```python
from build123d import *

# Parameters (mm, degrees)
RESSALTO_EXTRUS_O1_DEPTH = 6
ESBO_O7_W                = 6
ESBO_O7_H                = 39
CORTE_EXTRUS_O5_DEPTH    = 441.818556778
ESBO_O2_W                = 98
ESBO_O2_H                = 88
CORTE_EXTRUS_O1_DEPTH    = 10
FILETE2_R                = 12
CORTE_EXTRUS_O3_DEPTH    = 441.818556778
ESBO_O6_W                = 30
ESBO_O6_H                = 20
CORTE_EXTRUS_O4_DEPTH    = 441.818556778
FILETE3_START            = -1
FILETE3_DEPTH            = 8
FILETE3_2_DEPTH          = 6
ESBO_O8_W                = 6
ESBO_O8_H                = 34
RESSALTO_EXTRUS_O2_DEPTH = 31.4
ESBO_O9_W                = 25.4
ESBO_O9_H                = 55
RESSALTO_EXTRUS_O3_DEPTH = 6
CHANFRO1_SIZE            = 3
ESBO_O10_R               = 3.257801974
ESBO_O10_R_2             = 3
ESBO_O10_R_3             = 3.08509383
CORTE_EXTRUS_O6_DEPTH    = 463.399134947
FILETE4_R                = 5
ESBO_O11_W               = 402.172610053
ESBO_O11_H               = 13.658923547
CORTE_EXTRUS_O7_DEPTH    = 463.399134947
FILETE5_R                = 5


with BuildPart() as part:
    # Esboço1 → Ressalto-extrusão1 (new body)
    with BuildSketch(Plane.XY):
        Polygon((0, 94), (0, 238), (365, 238), (365, 94), (371, 94), (371, 0), (365, 0), (0, 0), (-6, 0), (-6, 94), align=None)
    extrude(amount=RESSALTO_EXTRUS_O1_DEPTH)

    # Esboço7 → Corte-extrusão5 (cut, through all)
    with BuildSketch(Plane.XY.offset(6)):
        with Locations((368, 19.5)):
            Rectangle(ESBO_O7_W, ESBO_O7_H)
        with Locations((-3, 19.5)):
            Rectangle(ESBO_O7_W, ESBO_O7_H)
    extrude(amount=-CORTE_EXTRUS_O5_DEPTH, mode=Mode.SUBTRACT)

    # Esboço2 → Corte-extrusão1 (cut)
    with BuildSketch(Plane.XY.offset(6)):
        with Locations((64, 144)):
            Rectangle(ESBO_O2_W, ESBO_O2_H)
        with Locations((301, 144)):
            Rectangle(ESBO_O2_W, ESBO_O2_H)
    extrude(amount=-CORTE_EXTRUS_O1_DEPTH, mode=Mode.SUBTRACT)

    # Filete2
    filete2_edges = [part.edges().sort_by_distance(p)[0] for p in [
        (15, 100, 3),
        (15, 188, 3),
        (113, 188, 3),
        (113, 100, 3),
        (350, 188, 3),
        (350, 100, 3),
        (252, 100, 3),
        (252, 188, 3),
    ]]
    fillet(filete2_edges, radius=FILETE2_R)

    # Esboço5 → Corte-extrusão3 (cut, through all)
    with BuildSketch(Plane.XY.offset(6)):
        with BuildLine():
            Line((183.428625358, 61.017420231), (160.787066224, 38.375861098))
            ThreePointArc((160.787066224, 38.375861098), (157.965710167, 37.207217155), (155.14435411, 38.375861098))
            Line((155.14435411, 38.375861098), (155.130211974, 38.390003233))
            ThreePointArc((155.130211974, 38.390003233), (153.961568031, 41.21135929), (155.130211974, 44.032715347))
            Line((155.130211974, 44.032715347), (177.771771108, 66.674274481))
            ThreePointArc((177.771771108, 66.674274481), (180.593127165, 67.842918424), (183.414483222, 66.674274481))
            Line((183.414483222, 66.674274481), (183.428625358, 66.660132345))
            ThreePointArc((183.428625358, 66.660132345), (184.597269301, 63.838776288), (183.428625358, 61.017420231))
        make_face()
        with BuildLine():
            Line((177.771771108, 82.046857483), (177.757628972, 82.032715347))
            ThreePointArc((177.757628972, 82.032715347), (176.588985029, 79.21135929), (177.757628972, 76.390003233))
            Line((177.757628972, 76.390003233), (200.399188106, 53.7484441))
            ThreePointArc((200.399188106, 53.7484441), (203.220544163, 52.579800157), (206.04190022, 53.7484441))
            Line((206.04190022, 53.7484441), (206.056042356, 53.762586235))
            ThreePointArc((206.056042356, 53.762586235), (207.224686299, 56.583942292), (206.056042356, 59.405298349))
            Line((206.056042356, 59.405298349), (183.414483222, 82.046857483))
            ThreePointArc((183.414483222, 82.046857483), (180.593127165, 83.215501426), (177.771771108, 82.046857483))
        make_face()
        with BuildLine():
            Line((183.428625358, 99.017420231), (160.787066224, 76.375861098))
            ThreePointArc((160.787066224, 76.375861098), (157.965710167, 75.207217155), (155.14435411, 76.375861098))
            Line((155.14435411, 76.375861098), (155.130211974, 76.390003233))
            ThreePointArc((155.130211974, 76.390003233), (153.961568031, 79.21135929), (155.130211974, 82.032715347))
            Line((155.130211974, 82.032715347), (177.771771108, 104.674274481))
            ThreePointArc((177.771771108, 104.674274481), (180.593127165, 105.842918424), (183.414483222, 104.674274481))
            Line((183.414483222, 104.674274481), (183.428625358, 104.660132345))
            ThreePointArc((183.428625358, 104.660132345), (184.597269301, 101.838776288), (183.428625358, 99.017420231))
        make_face()
        with BuildLine():
            Line((177.771771108, 120.046857483), (177.757628972, 120.032715347))
            ThreePointArc((177.757628972, 120.032715347), (176.588985029, 117.21135929), (177.757628972, 114.390003233))
            Line((177.757628972, 114.390003233), (200.399188106, 91.7484441))
            ThreePointArc((200.399188106, 91.7484441), (203.220544163, 90.579800157), (206.04190022, 91.7484441))
            Line((206.04190022, 91.7484441), (206.056042356, 91.762586235))
            ThreePointArc((206.056042356, 91.762586235), (207.224686299, 94.583942292), (206.056042356, 97.405298349))
            Line((206.056042356, 97.405298349), (183.414483222, 120.046857483))
            ThreePointArc((183.414483222, 120.046857483), (180.593127165, 121.215501426), (177.771771108, 120.046857483))
        make_face()
        with BuildLine():
            Line((183.428625358, 137.017420231), (160.787066224, 114.375861098))
            ThreePointArc((160.787066224, 114.375861098), (157.965710167, 113.207217155), (155.14435411, 114.375861098))
            Line((155.14435411, 114.375861098), (155.130211974, 114.390003233))
            ThreePointArc((155.130211974, 114.390003233), (153.961568031, 117.21135929), (155.130211974, 120.032715347))
            Line((155.130211974, 120.032715347), (177.771771108, 142.674274481))
            ThreePointArc((177.771771108, 142.674274481), (180.593127165, 143.842918424), (183.414483222, 142.674274481))
            Line((183.414483222, 142.674274481), (183.428625358, 142.660132345))
            ThreePointArc((183.428625358, 142.660132345), (184.597269301, 139.838776288), (183.428625358, 137.017420231))
        make_face()
        with BuildLine():
            Line((177.771771108, 158.046857483), (177.757628972, 158.032715347))
            ThreePointArc((177.757628972, 158.032715347), (176.588985029, 155.21135929), (177.757628972, 152.390003233))
            Line((177.757628972, 152.390003233), (200.399188106, 129.7484441))
            ThreePointArc((200.399188106, 129.7484441), (203.220544163, 128.579800157), (206.04190022, 129.7484441))
            Line((206.04190022, 129.7484441), (206.056042356, 129.762586235))
            ThreePointArc((206.056042356, 129.762586235), (207.224686299, 132.583942292), (206.056042356, 135.405298349))
            Line((206.056042356, 135.405298349), (183.414483222, 158.046857483))
            ThreePointArc((183.414483222, 158.046857483), (180.593127165, 159.215501426), (177.771771108, 158.046857483))
        make_face()
        with BuildLine():
            Line((183.428625358, 175.017420231), (160.787066224, 152.375861098))
            ThreePointArc((160.787066224, 152.375861098), (157.965710167, 151.207217155), (155.14435411, 152.375861098))
            Line((155.14435411, 152.375861098), (155.130211974, 152.390003233))
            ThreePointArc((155.130211974, 152.390003233), (153.961568031, 155.21135929), (155.130211974, 158.032715347))
            Line((155.130211974, 158.032715347), (177.771771108, 180.674274481))
            ThreePointArc((177.771771108, 180.674274481), (180.593127165, 181.842918424), (183.414483222, 180.674274481))
            Line((183.414483222, 180.674274481), (183.428625358, 180.660132345))
            ThreePointArc((183.428625358, 180.660132345), (184.597269301, 177.838776288), (183.428625358, 175.017420231))
        make_face()
    extrude(amount=-CORTE_EXTRUS_O3_DEPTH, mode=Mode.SUBTRACT)

    # Esboço6 → Corte-extrusão4 (cut, through all)
    with BuildSketch(Plane.XY.offset(6)):
        with Locations((107.5, 10)):
            Rectangle(ESBO_O6_W, ESBO_O6_H)
        with Locations((257.5, 10)):
            Rectangle(ESBO_O6_W, ESBO_O6_H)
    extrude(amount=-CORTE_EXTRUS_O4_DEPTH, mode=Mode.SUBTRACT)

    # Filete3: read off the stored shape, not the designer's step
    # Filete3 outline → Filete3 (cut)
    with BuildSketch(Plane.XY.offset(FILETE3_START)):
        with BuildLine():
            ThreePointArc((282.5, 0), (275.428932188, 2.928932188), (272.5, 10))
            Line((272.5, 10), (272.5, 0))
            Line((272.5, 0), (282.5, 0))
        make_face()
        with BuildLine():
            Line((92.5, 0), (92.5, 10))
            ThreePointArc((92.5, 10), (89.571067812, 2.928932188), (82.5, 0))
            Line((82.5, 0), (92.5, 0))
        make_face()
        with BuildLine():
            Line((122.5, 0), (132.5, 0))
            ThreePointArc((132.5, 0), (125.428932188, 2.928932188), (122.5, 10))
            Line((122.5, 10), (122.5, 0))
        make_face()
        with BuildLine():
            Line((242.5, 0), (242.5, 10))
            ThreePointArc((242.5, 10), (239.571067812, 2.928932188), (232.5, 0))
            Line((232.5, 0), (242.5, 0))
        make_face()
    extrude(amount=FILETE3_DEPTH, mode=Mode.SUBTRACT)

    # Filete3 2 outline → Filete3 2 (add)
    with BuildSketch(Plane.XY):
        with BuildLine():
            Line((272.5, 20), (262.5, 20))
            ThreePointArc((262.5, 20), (269.571067812, 17.071067812), (272.5, 10))
            Line((272.5, 10), (272.5, 20))
        make_face()
        with BuildLine():
            ThreePointArc((92.5, 10), (95.428932188, 17.071067812), (102.5, 20))
            Line((102.5, 20), (92.5, 20))
            Line((92.5, 20), (92.5, 10))
        make_face()
        with BuildLine():
            ThreePointArc((112.5, 20), (119.571067812, 17.071067812), (122.5, 10))
            Line((122.5, 10), (122.5, 20))
            Line((122.5, 20), (112.5, 20))
        make_face()
        with BuildLine():
            ThreePointArc((242.5, 10), (245.428932188, 17.071067812), (252.5, 20))
            Line((252.5, 20), (242.5, 20))
            Line((242.5, 20), (242.5, 10))
        make_face()
    extrude(amount=FILETE3_2_DEPTH)

    # Esboço8 → Ressalto-extrusão2 (add)
    with BuildSketch(Plane(origin=(365, 0, 0), x_dir=(0, 0, -1), z_dir=(1, 0, 0))):
        with Locations((-3, 207.827931833)):
            Rectangle(ESBO_O8_W, ESBO_O8_H)
    ressalto_extrus_o2 = extrude(amount=RESSALTO_EXTRUS_O2_DEPTH)

    # Espelhar1: Ressalto-extrusão2 across plane
    add(ressalto_extrus_o2.mirror(Plane.ZY.offset(-182.5)))

    # Esboço9 → Ressalto-extrusão3 (add, through all)
    with BuildSketch(Plane.XY.offset(6)):
        with Locations((383.7, 66.5)):
            Rectangle(ESBO_O9_W, ESBO_O9_H)
        with Locations((-18.7, 66.5)):
            Rectangle(ESBO_O9_W, ESBO_O9_H)
    extrude(amount=-RESSALTO_EXTRUS_O3_DEPTH)

    # Chanfro1
    chanfro1_edges = [part.edges().sort_by_distance(p)[0] for p in [
        (396.4, 224.827931833, 3),
        (396.4, 190.827931833, 3),
        (-31.4, 224.827931833, 3),
        (-31.4, 190.827931833, 3),
        (396.4, 94, 3),
        (396.4, 39, 3),
        (-31.4, 39, 3),
        (-31.4, 94, 3),
    ]]
    chamfer(chanfro1_edges, length=CHANFRO1_SIZE)

    # Esboço10 → Corte-extrusão6 (cut, through all)
    with BuildSketch(Plane.XY.offset(6)):
        with Locations((385.342976088, 207.820691694)):
            Circle(ESBO_O10_R)
        with Locations((385.3, 83.913025663)):
            Circle(ESBO_O10_R_2)
        with Locations((385.3, 49.913025663)):
            Circle(ESBO_O10_R_3)
        with Locations(Location((-20.3, 49.913025663, 0), (0, 0, 180))):
            Circle(ESBO_O10_R_3)
        with Locations(Location((-20.3, 83.913025663, 0), (0, 0, 180))):
            Circle(ESBO_O10_R_2)
        with Locations(Location((-20.342976088, 207.820691694, 0), (0, 0, 180))):
            Circle(ESBO_O10_R)
    extrude(amount=-CORTE_EXTRUS_O6_DEPTH, mode=Mode.SUBTRACT)

    # Filete4
    filete4_edges = [part.edges().sort_by_distance(p)[0] for p in [
        (365, 0, 3),
        (0, 0, 3),
    ]]
    fillet(filete4_edges, radius=FILETE4_R)

    # Esboço11 → Corte-extrusão7 (cut, through all)
    with BuildSketch(Plane.XY.offset(6)):
        with Locations((201.086305027, 2.170538226)):
            Rectangle(ESBO_O11_W, ESBO_O11_H)
    extrude(amount=-CORTE_EXTRUS_O7_DEPTH, mode=Mode.SUBTRACT)

    # Filete5
    filete5_edges = [part.edges().sort_by_distance(p)[0] for p in [
        (0, 9, 3),
        (122.550125629, 9, 3),
        (92.449874371, 9, 3),
        (242.449874371, 9, 3),
        (272.550125629, 9, 3),
        (365, 9, 3),
    ]]
    fillet(filete5_edges, radius=FILETE5_R)


solid = part.part
```
CAD build for the part. Positions are in the model's coordinates, mm. A direction names the side the tool comes from. Coordinates: 2 decimals unless noted, no trailing zeros. Order: outer loops, then holes, each group sorted by start corner. A loop starts at its lowest first (then second) coordinate and runs counter-clockwise, first axis right, second up. Notation, with made-up numbers: M 18.25,-29.5 L 64.25,-29.5 A17 ccw 64.25,-18.5 Z; hole C 50,62 d1. An arc over 180 degrees is marked long. Write each question's results on one line, items separated by ' | '. Start each with the question number.
Q1. Drill centre lines: probe 1 along Y at (x, z) = (277, 5.25); probe 2 along X at (y, z) = (102.5, 1.5); probe 3 along Y at (x, z) = (385.3, 1.55). Where is each one in solid material? Low to high. Write a range as from..to.
Q2. Cut at B-B (z = 3.75). Count the separate pieces of the cut face and the enclosed holes in it, then the cut area to 3 significant figures.
Q3. Flat gauge pins, fed straight in: P1, Ø3, axis at y = 228.5, z = 3, coming from the +X side; P2, Ø1.8, axis at x = 108.5, z = 3.5, coming from the -Y side; P3, Ø3, axis at y = 20.5, z = 4, coming from the -X side. Where does each tip first touch, or does it go through?
Q4. Cut at A-A (x = 300). List the corners of the cut face in (y, z), then the cut area to 3 significant figures.
Q5. Pull direction Y, two halves, no side cores. Call faces 4 (the cylindrical face through (96.37, 17.9, 2.96)), 5 (the flat face through (194.89, 70.57, 3.04)), 6 (the flat face through (180, 125, 6)): +Y half, -Y half, draft (parallel to the pull), parting line (faces both ways), or undercut.
Q6. Which spindle directions (+Z, -Z, +X, -X, +Y, -Y) get a long thin tool onto all of the face, cutting with end or side? Do faces 1 (the cylindrical face through (268.5, 18, 3)), 2 (the flat face through (180, 125, 0)), 3 (the flat face through (194.89, 146.57, 3.04)). Say none if no direction does.
Found:
1) probe 1: 9..100, 188..238 | probe 2: 0..19.67, 108.33..175.6, 184.54..189.65, 200.96..256.67, 345.33..365 | probe 3: 39..46.83, 53..80.91, 86.91..94, 190.83..204.56, 211.08..224.83
2) separate pieces: 1 | enclosed holes: 15 | area: 69,200 mm²
3) P1: x = 365 | P2: y = 20 | P3: x = 0
4) outline: M 9,0 L 100,0 L 100,6 L 9,6 Z; M 188,0 L 238,0 L 238,6 L 188,6 Z | area: 846 mm²
5) face 4: -Y half | face 5: undercut | face 6: draft
6) face 1: +Z, -Z, -Y | face 2: -Z, +X, -X, +Y, -Y | face 3: +Z, -Z
